Solid Edge part; units mm, degrees
sketch "Sketch1" plane through (0, 0, 0) normal (0, 0, 1) x (1, 0, 0)
  line L0 (210.2672, -0.1578) -> (210.2672, 144.8422)
  line L1 (210.2672, 144.8422) -> (0.2672, 144.8422)
  line L2 (0.2672, 144.8422) -> (0.2672, -0.1578)
  line L3 (0.2672, -0.1578) -> (210.2672, -0.1578)
extrude "Protrusion1" add sketch "Sketch1" along normal blind 5
hole "Hole_3" at (52.1036, 136.9518, 5) direction (0, 0, -1) diameter 3.2 depth 50.8
hole "Hole1" at (146.8525, 136.9518, 5) direction (0, 0, -1) diameter 3.2 depth 50.8
hole "Hole2" at (146.8195, 80.1518, 5) direction (0, 0, -1) diameter 3.2 depth 50.8
hole "Hole3" at (52.0525, 80.1518, 5) direction (0, 0, -1) diameter 3.2 depth 50.8
sketch "Sketch2" plane through (105.2672, 72.3422, 5) normal (0, 0, 1) x (1, 0, 0)
  line L0 (-54.5647, 16.2096) -> (42.9353, 16.2096)
  line L1 (42.9353, 16.2096) -> (42.9353, 56.2096)
  line L2 (42.9353, 56.2096) -> (-54.5647, 56.2096)
  line L3 (-54.5647, 56.2096) -> (-54.5647, 16.2096)
extrude "ExtrudedCutout_1" cut sketch "Sketch2" against normal blind 5
sketch "Sketch3" plane through (105.2672, 72.3422, 5) normal (0, 0, 1) x (1, 0, 0)
  circle A0 centre (86.9559, -57.0896) radius 6.15
extrude "ExtrudedCutout_2" cut sketch "Sketch3" against normal blind 5
sketch "Sketch4" plane through (105.2672, 72.3422, 5) normal (0, 0, 1) x (1, 0, 0)
  circle A0 centre (65.5473, -57.8825) radius 6.25
extrude "ExtrudedCutout_3" cut sketch "Sketch4" against normal blind 5
sketch "Sketch5" plane through (105.2672, 72.3422, 5) normal (0, 0, 1) x (1, 0, 0)
  circle A0 centre (75.3266, -43.0815) radius 3.5
extrude "ExtrudedCutout_4" cut sketch "Sketch5" against normal blind 5
hole "Hole_7" at (66.6096, 57.7955, 5) direction (0, 0, -1) diameter 3.2 depth 50.8
hole "Hole_8" at (66.7973, 28.6755, 5) direction (0, 0, -1) diameter 3.2 depth 50.8
sketch "Sketch6" plane through (105.2672, 72.3422, 5) normal (0, 0, 1) x (1, 0, 0)
  line L0 (-53.8048, -45.5734) -> (-53.8048, -12.5734)
  line L1 (-53.8048, -12.5734) -> (-86.8048, -12.5734)
  line L2 (-86.8048, -12.5734) -> (-86.8048, -45.5734)
  line L3 (-86.8048, -45.5734) -> (-53.8048, -45.5734)
extrude "ExtrudedCutout_5" cut sketch "Sketch6" against normal blind 5
sketch "Sketch7" plane through (105.2672, 72.3422, 5) normal (0, 0, 1) x (1, 0, 0)
  circle A0 centre (72.9478, 48.3676) radius 6.25
  circle A1 centre (72.9478, 48.3676) radius 6.25
extrude "ExtrudedCutout_6" cut sketch "Sketch7" against normal blind 5
sketch "Sketch8" plane through (105.2672, 72.3422, 5) normal (0, 0, 1) x (1, 0, 0)
  circle A0 centre (73.4765, 21.6729) radius 6.25
extrude "ExtrudedCutout_7" cut sketch "Sketch8" against normal blind 5
sketch "Sketch9" plane through (105.2672, 72.3422, 5) normal (0, 0, 1) x (1, 0, 0)
  circle A0 centre (73.7408, -6.8719) radius 6.25
extrude "ExtrudedCutout_8" cut sketch "Sketch9" against normal blind 5
sketch "Sketch10" plane through (105.2672, 72.3422, 5) normal (0, 0, 1) x (1, 0, 0)
  circle A0 centre (6.079, -29.0734) radius 11.5
extrude "ExtrudedCutout_10" cut sketch "Sketch10" against normal blind 5
sketch "Sketch11" plane through (105.2672, 72.3422, 5) normal (0, 0, 1) x (1, 0, 0)
  circle A0 centre (-13.4795, -54.9752) radius 2
extrude "ExtrudedCutout_11" cut sketch "Sketch11" against normal blind 5
hole "Hole_11" at (94.4307, 43.2688, 5) direction (0, 0, -1) diameter 3.2 depth 50.8
hole "Hole4" at (127.733, 43.2688, 5) direction (0, 0, -1) diameter 3.2 depth 50.8
hole "Hole_13" at (2.7672, 142.0476, 5) direction (0, 0, -1) diameter 3.2 depth 50.8
hole "Hole5" at (207.7672, 142.0476, 5) direction (0, 0, -1) diameter 3.2 depth 50.8
hole "Hole6" at (207.7672, 2.0476, 5) direction (0, 0, -1) diameter 3.2 depth 50.8
hole "Hole7" at (2.7672, 2.0476, 5) direction (0, 0, -1) diameter 3.2 depth 50.8
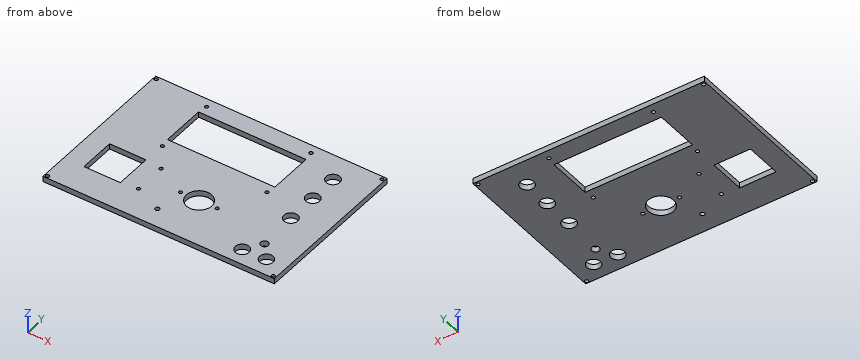
Here's how the part is built. I have some questions about the finished solid (model axes, mm). Give positions to 0.01 mm unless a question says otherwise; leave off trailing zeros. Order: outer loops, then holes, each group sorted by start corner. A loop starts at its lowest first (then second) coordinate and runs counter-clockwise, first axis right, second up. Notation, with made-up numbers: (54.5, 1.5) - (79.5, 1.5) arc R19 ccw to (79.5, 8.5) - close; hole circle Ø3 at (31.5, 19). An arc over 180 degrees is marked (long way). Answer as a JSON object with one key per item and string values. Group by question number.
Item 1: If we section it at A-A on x = 71.5: Please give me the cut outline in (y, z), and give its area (3 significant figures).
Item 2: If we section it at C-C on x = 111.5: Please give me the cut outline in (y, z), and give its area (3 significant figures).
Item 3: If we section it at B-B on y = 107.5: Please give me the cut outline in (x, z), and give its area (4 significant figures).
Item 4: If we section it at D-D on z = 2.75: Give the number of separate pieces and of enclosed holes in the cut face, and give its area (3 significant figures).
Item 5: Please list where these lines run through material, in increasing order: probe 1 along Y at (x, z) = (128, 4.4); probe 2 along X at (y, z) = (98, 3.5); probe 3 along Y at (x, z) = (103, 1.35).
Result set:
{
 "1": {"outline": "(-0.16, 0) - (88.55, 0) - (88.55, 5) - (-0.16, 5) - close; (128.55, 0) - (144.84, 0) - (144.84, 5) - (128.55, 5) - close", "area": "525 mm²"},
 "2": {"outline": "(-0.16, 0) - (31.77, 0) - (31.77, 5) - (-0.16, 5) - close; (54.77, 0) - (88.55, 0) - (88.55, 5) - (54.77, 5) - close; (128.55, 0) - (144.84, 0) - (144.84, 5) - (128.55, 5) - close", "area": "410 mm²"},
 "3": {"outline": "(0.27, 0) - (50.7, 0) - (50.7, 5) - (0.27, 5) - close; (148.2, 0) - (210.27, 0) - (210.27, 5) - (148.2, 5) - close", "area": "562.5 mm²"},
 "4": {"separate pieces": "1", "enclosed holes": "22", "area": "24,300 mm²"},
 "5": {"probe 1": "-0.16 to 41.69, 44.85 to 88.55, 128.55 to 144.84", "probe 2": "0.27 to 50.7, 148.2 to 173.93, 183.56 to 210.27", "probe 3": "-0.16 to 35.36, 51.18 to 88.55, 128.55 to 144.84"}
}
